```python
from build123d import *

# Parameters (mm, degrees)
SKETCH1_W            = 24
SKETCH1_H            = 26
BOSS_EXTRUDE1_DEPTH  = 24
SKETCH2_R            = 2.7
BOSS_EXTRUDE2_DEPTH  = 9
FILLET2_R            = 2.7
FILLET2_OF_MIRROR2_R = 2.7


with BuildPart() as part:
    # Sketch1 → Boss-Extrude1 (new body)
    with BuildSketch(Plane(origin=(0, 0, 0), x_dir=(1, 0, 0), z_dir=(0, 1, 0))):
        Rectangle(SKETCH1_W, SKETCH1_H)
    extrude(amount=BOSS_EXTRUDE1_DEPTH)

    # Sketch2 → Boss-Extrude2 (add)
    with BuildSketch(Plane.ZY.offset(12)):
        with Locations((-4.5, 7.148873243)):
            Circle(SKETCH2_R)
    boss_extrude2 = extrude(amount=BOSS_EXTRUDE2_DEPTH)

    # Fillet2
    fillet2_edges = [part.edges().sort_by_distance(p)[0] for p in [
        (-21, 7.148873243, -7.2),
    ]]
    fillet(fillet2_edges, radius=FILLET2_R)

    # Mirror2: Boss-Extrude2 across plane
    add(boss_extrude2.mirror(Plane.XY))

    # Fillet2 of Mirror2
    fillet2_of_mirror2_edges = [part.edges().sort_by_distance(p)[0] for p in [
        (-21, 7.148873243, 7.2),
    ]]
    fillet(fillet2_of_mirror2_edges, radius=FILLET2_OF_MIRROR2_R)


solid = part.part
```
The listing builds one solid part. Answer for the finished solid, in the listing's coordinates (mm). Give positions to 0.01 mm unless a question says otherwise; leave off trailing zeros. Loops run counter-clockwise (first coordinate to the right, second up) from the corner with the lowest first, then second, coordinate; pieces in that order, holes last. Notation, with made-up numbers: (-13, -33.5) - (42, -33.5) arc R31 ccw to (42, 1.5) - close; hole circle Ø4 at (20.25, 46). An arc over 180 degrees is marked (long way). Return JSON: item names as keys, results as strings. Group by question number.
1. Find section C-C (x = -14). Write down the section's boundary in (y, z), then the cut area to 3 significant figures.
2. Given pin 1 Ø1 at (y, z) = (2.5, 4.5) entering from -X, flat-ended and moving along its own axis, determine where the tip first touches the part or whether it passes through.
3. Determine the mould class of faces 1 (the flat face through (0, 12, -13)), 2 (the cylindrical face through (-15.106, 9.826, -4.851)), 3 (the cylindrical face through (-15.106, 9.826, 4.851)), 4 (the flat face through (0, 12, 13)) for opening direction Z: pulls with the +Z half, pulls with the -Z half, needs draft (parallel to the pull), parting line crosses it, or undercut.
4. Find section B-B (y = 19.5). Write down the section's boundary in (x, z), then the cut area to 3 significant figures.
5. Find section D-D (z = 8.5). Write down the section's boundary in (x, y), then the cut area to 3 significant figures.
6. Straight lines are drawn through the part: line 1 (X direction, y = 1, z = 10.5); line 2 (Y direction, x = -19.5, z = 3). For each, find the intervals that lie inside material, in ascending order. Write a range as [from, to].
7. Find section A-A (z = -4.5). Write down the section's boundary in (x, y).
Verdict:
{
 "1": {"outline": "circle Ø5.4 at (7.15, -4.5); circle Ø5.4 at (7.15, 4.5)", "area": "45.8 mm^2"},
 "2": {"pin 1": "stops at x = -12"},
 "3": {"face 1": "pulls with the -Z half", "face 2": "undercut", "face 3": "undercut", "face 4": "pulls with the +Z half"},
 "4": {"outline": "(-12, -13) - (12, -13) - (12, 13) - (-12, 13) - close", "area": "624 mm^2"},
 "5": {"outline": "(-12, 0) - (12, 0) - (12, 24) - (-12, 24) - close", "area": "576 mm^2"},
 "6": {"line 1": "x = [-12, 12]", "line 2": "y = [5.25, 9.05]"},
 "7": {"outline": "(-18.3, 4.45) - (-12, 4.45) - (-12, 0) - (12, 0) - (12, 24) - (-12, 24) - (-12, 9.85) - (-18.3, 9.85) arc R2.7 ccw to start"}
}
